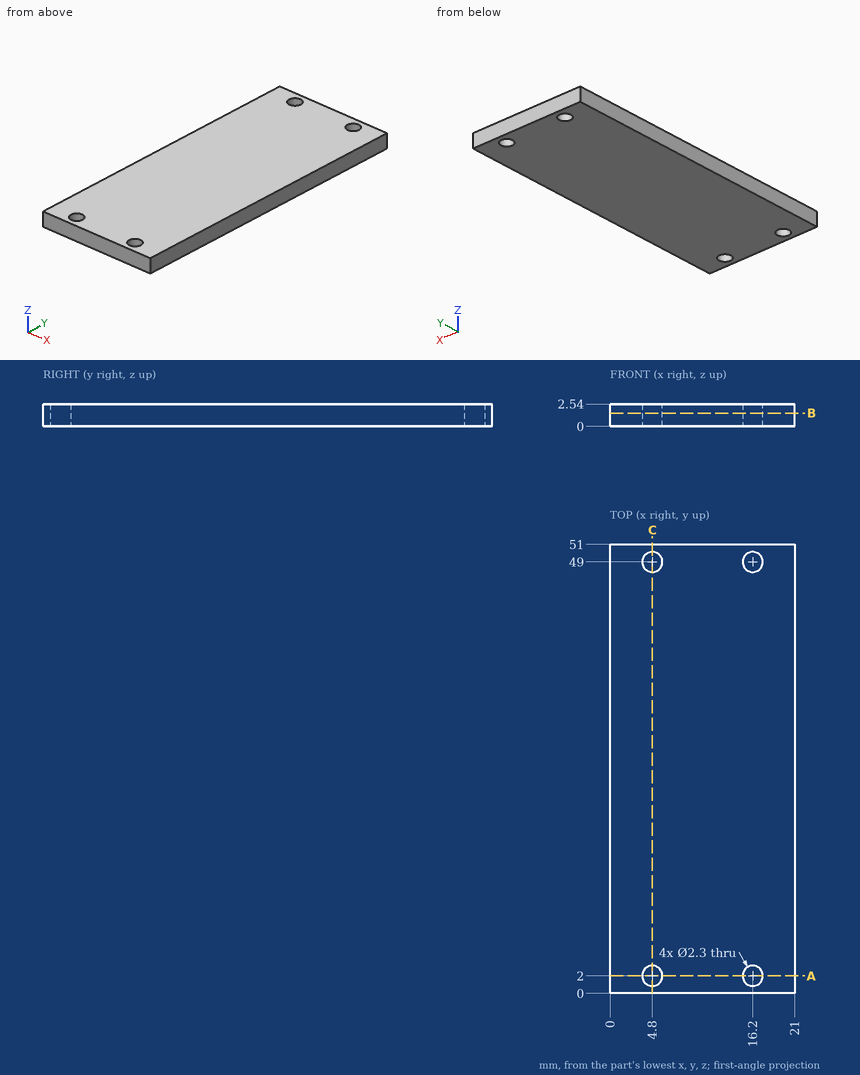
Verification items for this drawing (mm, ordinates from the low corner). Coordinates: 2 decimals unless noted, no trailing zeros. Order: outer loops, then holes, each group sorted by start corner. A loop starts at its lowest first (then second) coordinate and runs counter-clockwise, first axis right, second up. Notation, with made-up numbers: (23.25, 4.25) - (82.25, 4.25) arc R18 ccw to (82.25, 27.25) - close; hole circle Ø6 at (0, -36.75). An arc over 180 degrees is marked (long way). Answer as a JSON object with one key per item and string values. Group by question number.
Item 1: Depth check by flat-ended pin: pin 1 Ø1.4 at (x, y) = (16.2, 2) entering from -Z. Enter the tip coordinate at first touch or a pass-through.
Item 2: Sectioned sample at C-C, the plane x = 4.8. Record the cut outline in (y, z), and give its area (3 significant figures).
Item 3: Sectioned sample at A-A, the plane y = 2. Record the cut outline in (x, z), and give its area (3 significant figures).
Item 4: Sectioned sample at B-B, the plane z = 1.5. Record the cut outline in (x, y).
Item 5: Scan lines: probe 1 along Y at (x, z) = (4.8, 1.8); probe 2 along Y at (x, z) = (17, 0.1). Record each from-to range of solid material in increasing order.
Resolved:
{
 "1": {"pin 1": "through"},
 "2": {"outline": "(0, 0) - (0.85, 0) - (0.85, 2.54) - (0, 2.54) - close; (3.15, 0) - (47.85, 0) - (47.85, 2.54) - (3.15, 2.54) - close; (50.15, 0) - (51, 0) - (51, 2.54) - (50.15, 2.54) - close", "area": "118 mm^2"},
 "3": {"outline": "(0, 0) - (3.65, 0) - (3.65, 2.54) - (0, 2.54) - close; (5.95, 0) - (15.05, 0) - (15.05, 2.54) - (5.95, 2.54) - close; (17.35, 0) - (21, 0) - (21, 2.54) - (17.35, 2.54) - close", "area": "41.7 mm^2"},
 "4": {"outline": "(0, 0) - (21, 0) - (21, 51) - (0, 51) - close; hole circle Ø2.3 at (4.8, 2); hole circle Ø2.3 at (4.8, 49); hole circle Ø2.3 at (16.2, 2); hole circle Ø2.3 at (16.2, 49)"},
 "5": {"probe 1": "0 to 0.85, 3.15 to 47.85, 50.15 to 51", "probe 2": "0 to 1.17, 2.83 to 48.17, 49.83 to 51"}
}
